Part model, mm, in its own coordinate system. A direction names the side the tool comes from. Round coordinates to 2 decimals unless told otherwise and drop trailing zeros. Loops run counter-clockwise (first coordinate to the right, second up) from the corner with the lowest first, then second, coordinate; pieces in that order, holes last. Notation, with made-up numbers: (64.25, 16) - (84.25, 16) arc R28 ccw to (84.25, 53) - close; hole circle Ø11 at (-26.5, 43). An arc over 180 degrees is marked (long way). Put each result on its own line as item: value.
from build123d import *

# Parameters (mm, degrees)
F0_R     = 0.4
F1_DEPTH = 2.5
F3_DEPTH = 35


with BuildPart() as f1:
    # F0 (on Front) → F1 (new body, symmetric)
    with BuildSketch(Plane.XZ):
        Polygon((0, 10.2), (-1, 10.2), (-1, -1), (4, -1), (4, -1.5), (7.2, -1.5), (7.8, -0.9), (8.4, -1.5), (9, -0.9), (16.7, -0.9), (16.7, -0.4), (18.7, -0.4), (18.7, 0.9), (9, 0.9), (8.4, 1.5), (7.8, 0.9), (7.2, 1.5), (4, 1.5), (4, 1), (1, 1), (1, 3.5), (0.8, 3.5), (0.8, 8), (0, 8), align=None)
        Circle(F0_R, mode=Mode.SUBTRACT)
        with Locations((13.7, 0)):
            Circle(F0_R, mode=Mode.SUBTRACT)
    extrude(amount=F1_DEPTH, both=True)

    # F2 (on Right) → F3 (intersect, symmetric)
    with BuildSketch(Plane.YZ):
        with BuildLine():
            ThreePointArc((0.935946, 3.802558), (0.992896, 3.952874), (0.999207, 4.113493))
            Line((0.999207, 4.113493), (0.251877, 10.2))
            Line((0.251877, 10.2), (-0.23447, 10.140284))
            Line((-0.23447, 10.140284), (0.492878, 4.216506))
            ThreePointArc((0.492878, 4.216506), (0.486568, 4.055888), (0.429618, 3.905572))
            Line((0.429618, 3.905572), (-0.566449, 2.180333))
            ThreePointArc((-0.566449, 2.180333), (-0.616399, 2.059743), (-0.633436, 1.930333))
            Line((-0.633436, 1.930333), (-0.633436, -1.5))
            Line((-0.633436, -1.5), (-0.143436, -1.5))
            Line((-0.143436, -1.5), (-0.143436, 1.799038))
            ThreePointArc((-0.143436, 1.799038), (-0.126399, 1.928448), (-0.076449, 2.049038))
            Line((-0.076449, 2.049038), (0.935946, 3.802558))
        make_face()
    extrude(amount=F3_DEPTH, both=True, mode=Mode.INTERSECT)


solid = f1.part
1. Two-plate mould, pull along X, no slides. Class faces 3 (the flat face through (0.8, 0.5, 5.7)), 4 (the flat face through (1, -0.09, 2.34)), 5 (the flat face through (9, -0.143, 0)): pulls with the +X half, pulls with the -X half, needs draft (parallel to the pull), parting line crosses it, or undercut.
A:
face 3: pulls with the +X half
face 4: undercut
face 5: needs draft
2. Band-saw the part on D-D (z = 3). List the corners of the cut face in (x, y).
A:
outline: (-1, -0.09) - (1, -0.09) - (1, 0.47) - (-1, 0.47) - close
3. Probe line 1 along X through (y, z) = (-0.3, 0); line 2 along Z through (x, y) = (13.7, -0.5); line 3 along Y through (x, z) = (16.25, 0). List the from-to ranges inside material, lowest first. Write a range as [from, to].
A:
line 1: x = [-1, -0.4], [0.4, 13.3], [14.1, 18.7]
line 2: z = [-0.9, -0.4], [0.4, 0.9]
line 3: y = [-0.63, -0.14]
4. Tool access for faces 1 (the flat face through (-0.1, 0.2, 6.6)), 2 (the flat face through (7, -0.633, 0)): list every direction of +Z, -Z, +X, -X, +Y, -Y with a clear straight run to the whole face (end or side of a thin tool).
A:
face 1: +X, -X, -Y
face 2: +Z, -Z, +X, -X, -Y
5. Band-saw the part on A-A (z = 0). List the corners of the cut face in (x, y).
A:
outline: (-1, -0.63) - (-0.4, -0.63) - (-0.4, -0.14) - (-1, -0.14) - close; (0.4, -0.63) - (13.3, -0.63) - (13.3, -0.14) - (0.4, -0.14) - close; (14.1, -0.63) - (18.7, -0.63) - (18.7, -0.14) - (14.1, -0.14) - close
6. Band-saw the part on B-B (x = 13.7). List the corners of the cut face in (y, z), plus the area to 3 significant figures.
A:
outline: (-0.63, -0.9) - (-0.14, -0.9) - (-0.14, -0.4) - (-0.63, -0.4) - close; (-0.63, 0.4) - (-0.14, 0.4) - (-0.14, 0.9) - (-0.63, 0.9) - close
area: 0.490 mm²
7. Pin check, flat tips, straight feed: P1, Ø0.5, axis at x = 17.5, y = -0.5, coming from the -Z side; P2, Ø0.5, axis at x = 1.5, y = -0.5, coming from the -Z side; P3, Ø5, axis at x = 14, z = 2, coming from the +Y side. Stop position of each tip, or through.
A:
P1: stops at z = -0.4
P2: stops at z = -1
P3: stops at y = -0.14
8. Band-saw the part on C-C (x = 7). List the corners of the cut face in (y, z).
A:
outline: (-0.63, -1.5) - (-0.14, -1.5) - (-0.14, 1.5) - (-0.63, 1.5) - close
